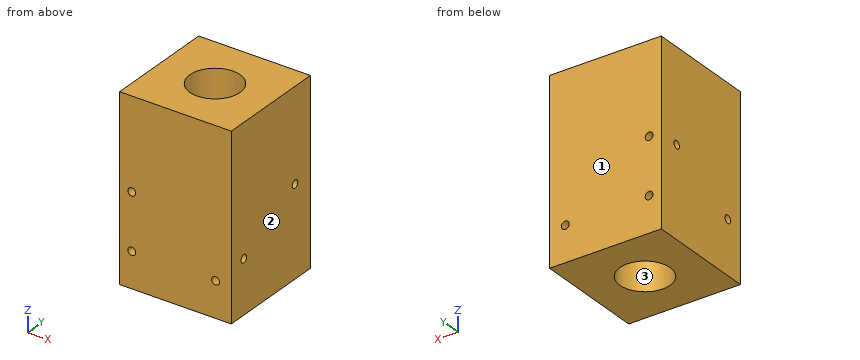
from build123d import *

# Parameters (mm, degrees)
SKETCH1_W           = 40
SKETCH1_H           = 40
SKETCH1_R           = 9
BOSS_EXTRUDE1_DEPTH = 65
SKETCH2_R           = 1.4
CUT_EXTRUDE1_DEPTH  = 41
SKETCH3_R           = 1.4
CUT_EXTRUDE2_DEPTH  = 65


with BuildPart() as part:
    # Sketch1 → Boss-Extrude1 (new body)
    with BuildSketch(Plane.XY):
        Rectangle(SKETCH1_W, SKETCH1_H)
        Circle(SKETCH1_R, mode=Mode.SUBTRACT)
    extrude(amount=BOSS_EXTRUDE1_DEPTH)

    # Sketch2 → Cut-Extrude1 (cut, through all)
    with BuildSketch(Plane(origin=(0, 20, 0), x_dir=(1, 0, 0), z_dir=(0, 1, 0))):
        with Locations((14.364756044, -12.672944901)):
            Circle(SKETCH2_R)
        with Locations((-15.635243956, -32.672944901)):
            Circle(SKETCH2_R)
        with Locations((-15.635243956, -12.672944901)):
            Circle(SKETCH2_R)
    extrude(amount=-CUT_EXTRUDE1_DEPTH, mode=Mode.SUBTRACT)

    # Sketch3 → Cut-Extrude2 (cut)
    with BuildSketch(Plane(origin=(20, 0, 0), x_dir=(0, 0, -1), z_dir=(1, 0, 0))):
        with Locations((-32.021199164, 12.205306236)):
            Circle(SKETCH3_R)
        with Locations((-19.021201071, -13.641280886)):
            Circle(SKETCH3_R)
    extrude(amount=-CUT_EXTRUDE2_DEPTH, mode=Mode.SUBTRACT)


solid = part.part
Work out the finished part from the listing and answer in its coordinate system (mm). Face numbers are marked on the shaded views. Round coordinates to 2 decimals unless told otherwise and drop trailing zeros. Loops run counter-clockwise (first coordinate to the right, second up) from the corner with the lowest first, then second, coordinate; pieces in that order, holes last. Notation, with made-up numbers: (57.5, 15.25) - (116.5, 15.25) arc R18 cw to (116.5, 49.25) - close; hole circle Ø9 at (-12, 79). An arc over 180 degrees is marked (long way). Use one line per item in the form item = value. Start each with the question number.
(1) A flat-ended cylindrical pin translates along its axis: P1, Ø4.5, axis at x = -15.64, z = 32.67, coming from the +Y side. Find the tip coordinate at first contact, or state that the pin passes through.
(2) Consider line 1 (Z direction, x = -16.5, y = -17.5); line 2 (Y direction, x = -4, z = 29.5); line 3 (Y direction, x = -4.5, z = 13). Determine where each line is inside the solid, lowest interval first.
(3) Find section A-A on x = 8. Determine the outline of the cut face in (y, z).
(4) Find section D-D on y = 0. Determine the outline of the cut face in (x, z).
(5) Find section C-C on z = 43.5. Determine the outline of the cut face in (x, y).
(6) Find section B-B on y = -6. Determine the outline of the cut face in (x, z), and give its area (3 significant figures).
(7) Determine the mould class of the marked faces 1, 2 and 3 for opening direction X: +X half, -X half, draft (parallel to the pull), parting line (faces both ways), or undercut.
Answer list:
q1.P1 = 20
q2.line_1 = 0 to 11.57, 13.77 to 31.57, 33.77 to 65
q2.line_2 = -20 to -8.06, 8.06 to 20
q2.line_3 = -20 to -7.79, 7.79 to 20
q3.outline = (-20, 0) - (-4.12, 0) - (-4.12, 65) - (-20, 65) - close; (4.12, 0) - (20, 0) - (20, 65) - (4.12, 65) - close; hole circle Ø2.8 at (-13.64, 19.02); hole circle Ø2.8 at (12.21, 32.02)
q4.outline = (-20, 0) - (-9, 0) - (-9, 65) - (-20, 65) - close; (9, 0) - (20, 0) - (20, 65) - (9, 65) - close; hole circle Ø2.8 at (-15.64, 12.67); hole circle Ø2.8 at (-15.64, 32.67); hole circle Ø2.8 at (14.36, 12.67)
q5.outline = (-20, -20) - (20, -20) - (20, 20) - (-20, 20) - close; hole circle Ø18 at (0, 0)
q6.outline = (-20, 0) - (-6.71, 0) - (-6.71, 65) - (-20, 65) - close; (6.71, 0) - (20, 0) - (20, 65) - (6.71, 65) - close; hole circle Ø2.8 at (-15.64, 12.67); hole circle Ø2.8 at (-15.64, 32.67); hole circle Ø2.8 at (14.36, 12.67)
q6.area = 1,710 mm^2
q7.face_1 = draft
q7.face_2 = +X half
q7.face_3 = undercut
